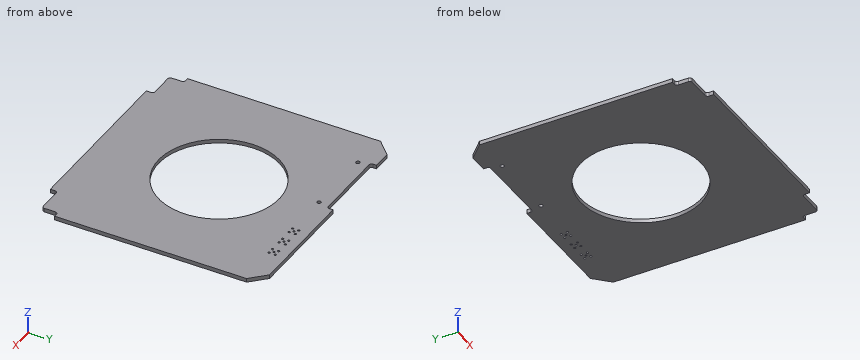
from build123d import *

# Parameters (mm, degrees)
SKETCH1_R           = 0.425
SKETCH1_R_2         = 25
SKETCH1_R_3         = 0.8
BOSS_EXTRUDE1_DEPTH = 1.6


with BuildPart() as part:
    # Sketch1 → Boss-Extrude1 (new body)
    with BuildSketch(Plane(origin=(0, 0, -0.0125), x_dir=(-1, 0, 0), z_dir=(0, 0, -1))):
        with BuildLine():
            Line((47.8, -40.8), (49.3, -40.8))
            Line((49.3, -40.8), (49.3, 39.2))
            Line((49.3, 39.2), (43.2, 45.3))
            Line((43.2, 45.3), (35.500000017, 45.3))
            Line((35.500000017, 45.3), (35.500000017, 43.8))
            ThreePointArc((35.500000017, 43.8), (35.207106799, 43.092893219), (34.500000017, 42.8))
            Line((34.500000017, 42.8), (4.500000014, 42.8))
            ThreePointArc((4.500000014, 42.8), (3.792893232, 43.092893219), (3.500000014, 43.8))
            Line((3.500000014, 43.8), (3.500000014, 45.3))
            Line((3.500000014, 45.3), (-43.2, 45.3))
            Line((-43.2, 45.3), (-49.3, 39.2))
            Line((-49.3, 39.2), (-49.3, -40.4))
            Line((-49.3, -40.4), (-47.8, -40.4))
            ThreePointArc((-47.8, -40.4), (-47.092893219, -40.692893219), (-46.8, -41.4))
            Line((-46.8, -41.4), (-46.8, -46))
            ThreePointArc((-46.8, -46), (-46.507106781, -46.707106781), (-45.8, -47))
            Line((-45.8, -47), (-36.3, -47))
            ThreePointArc((-36.3, -47), (-35.592893219, -47.292893219), (-35.3, -48))
            Line((-35.3, -48), (-35.3, -50))
            Line((-35.3, -50), (35.3, -50))
            Line((35.3, -50), (35.3, -48))
            ThreePointArc((35.3, -48), (35.592893219, -47.292893219), (36.3, -47))
            Line((36.3, -47), (45.8, -47))
            ThreePointArc((45.8, -47), (46.507106781, -46.707106781), (46.8, -46))
            Line((46.8, -46), (46.8, -41.8))
            ThreePointArc((46.8, -41.8), (47.092893219, -41.092893219), (47.8, -40.8))
        make_face()
        with Locations(Location((-13.87, 38.33, 0), (0, 0, 180))):
            Circle(SKETCH1_R, mode=Mode.SUBTRACT)
        Circle(SKETCH1_R_2, mode=Mode.SUBTRACT)
        with Locations(Location((-22.54, 39.6, 0), (0, 0, 180))):
            Circle(SKETCH1_R, mode=Mode.SUBTRACT)
        with Locations(Location((-23.81, 40.87, 0), (0, 0, 180))):
            Circle(SKETCH1_R, mode=Mode.SUBTRACT)
        with Locations(Location((-21.27, 40.87, 0), (0, 0, 180))):
            Circle(SKETCH1_R, mode=Mode.SUBTRACT)
        with Locations(Location((-13.87, 40.87, 0), (0, 0, 180))):
            Circle(SKETCH1_R, mode=Mode.SUBTRACT)
        with Locations(Location((-31.21, 40.87, 0), (0, 0, 180))):
            Circle(SKETCH1_R, mode=Mode.SUBTRACT)
        with Locations(Location((-16.41, 40.87, 0), (0, 0, 180))):
            Circle(SKETCH1_R, mode=Mode.SUBTRACT)
        with Locations(Location((-15.14, 39.6, 0), (0, 0, 180))):
            Circle(SKETCH1_R, mode=Mode.SUBTRACT)
        with Locations(Location((-29.94, 39.6, 0), (0, 0, 180))):
            Circle(SKETCH1_R, mode=Mode.SUBTRACT)
        with Locations(Location((-28.67, 40.87, 0), (0, 0, 180))):
            Circle(SKETCH1_R, mode=Mode.SUBTRACT)
        with Locations(Location((-28.67, 38.33, 0), (0, 0, 180))):
            Circle(SKETCH1_R, mode=Mode.SUBTRACT)
        with Locations(Location((-16.41, 38.33, 0), (0, 0, 180))):
            Circle(SKETCH1_R, mode=Mode.SUBTRACT)
        with Locations(Location((-21.27, 38.33, 0), (0, 0, 180))):
            Circle(SKETCH1_R, mode=Mode.SUBTRACT)
        with Locations(Location((-23.81, 38.33, 0), (0, 0, 180))):
            Circle(SKETCH1_R, mode=Mode.SUBTRACT)
        with Locations(Location((-31.21, 38.33, 0), (0, 0, 180))):
            Circle(SKETCH1_R, mode=Mode.SUBTRACT)
        with Locations((33.775, 38.54)):
            Circle(SKETCH1_R_3, mode=Mode.SUBTRACT)
        with Locations((5.225, 38.54)):
            Circle(SKETCH1_R_3, mode=Mode.SUBTRACT)
    extrude(amount=-BOSS_EXTRUDE1_DEPTH)


solid = part.part
Verification items for the finished model (mm, model axes). Coordinates: 2 decimals unless noted, no trailing zeros. Write each loop counter-clockwise with the first axis right and the second up, starting at its lowest first coordinate (ties: lowest second). Pieces come first, ordered by that corner, then holes. Notation, with made-up numbers: (46.25, -18) -> (82.25, -18) arc R20 cw to (82.25, 1) -> close; hole circle Ø11 at (84.5, -4). An arc over 180 degrees is marked (long way). One line per item, written item: value. Start each with the question number.
Q1. Cross-section at B-B on y = -9. Enter the section's corners in (x, z).
Q2. Thickness scan on L1, parallel to Y at x = 31.21, z = 0.5 (3 decimals); L2, parallel to Y at x = -0.5, z = 1.35 (3 decimals); L3, parallel to Y at x = 16.41, z = 1.1 (3 decimals). Record the ranges inside material, lowest first. Write a range as from..to.
Q3. Cross-section at A-A on x = -22.5. Enter the section's corners in (y, z).
Q4. Go/stop test with flat-tipped pins: P1, Ø0.8, axis at x = -48.5, z = 1, coming from the -Y side; P2, Ø0.8, axis at y = -44, z = 1, coming from the -X side; P3, Ø0.5, axis at x = -12.5, z = 1, coming from the +Y side; P4, Ø2.5, axis at x = -5.225, y = 38.54, coming from the -Z side. Record where each tip stops, or that it passes through.
Q5. Cross-section at C-C on z = 0.85. State how many separate pieces and enclosed holes the cut face has, and give its area (3 significant figures).
Checked values:
1. outline: (-49.3, -0.01) -> (-23.32, -0.01) -> (-23.32, 1.59) -> (-49.3, 1.59) -> close; (23.32, -0.01) -> (49.3, -0.01) -> (49.3, 1.59) -> (23.32, 1.59) -> close
2. L1: y = -50..37.905, 38.755..40.445, 41.295..45.3
2. L2: y = -50..-24.995, 24.995..45.3
2. L3: y = -50..-18.86, 18.86..37.905, 38.755..40.445, 41.295..45.3
3. outline: (-50, -0.01) -> (-10.9, -0.01) -> (-10.9, 1.59) -> (-50, 1.59) -> close; (10.9, -0.01) -> (42.8, -0.01) -> (42.8, 1.59) -> (10.9, 1.59) -> close
4. P1: stops at y = -40.8
4. P2: stops at x = -46.8
4. P3: stops at y = 42.8
4. P4: stops at z = -0.01
5. separate pieces: 1
5. enclosed holes: 18
5. area: 7,190 mm²
